Can you work these out from the model? Positions are in its coordinate system, mm. Face numbers are marked on the shaded views. A direction names the side the tool comes from. Give positions to 0.01 mm unless a question says otherwise; leave off trailing zeros. Loops run counter-clockwise (first coordinate to the right, second up) from the corner with the lowest first, then second, coordinate; pieces in that order, holes last. Notation, with made-up numbers: M -26,12.5 L -12,12.5 A26 cw -12,33.5 Z; hole C 22.25,2 d9. An arc over 180 degrees is marked long. Use CSV: the item, a comma, the result in double quotes.
from build123d import *

# Parameters (mm, degrees)
F0_W     = 50
F0_H     = 50
F1_DEPTH = 25
F2_R     = 12.5
F3_DEPTH = 50
F4_R     = 20
F5_DEPTH = 50


with BuildPart() as f1:
    # F0 (on Front) → F1 (new body, symmetric)
    with BuildSketch(Plane.XZ):
        Rectangle(F0_W, F0_H)
    extrude(amount=F1_DEPTH, both=True)

    # F2 (on face) → F3 (cut)
    with BuildSketch(Plane.XZ.offset(25)):
        Circle(F2_R)
    extrude(amount=-F3_DEPTH, mode=Mode.SUBTRACT)

    # F4 (on face) → F5 (join)
    with BuildSketch(Plane.XY.offset(25)):
        Circle(F4_R)
    extrude(amount=F5_DEPTH)

    # F6 (on Front) → F7 (revolve)
    with BuildSketch(Plane.XZ):
        Polygon((0, 103), (0, 75), (10, 75), align=None)
    revolve(axis=Axis((0, 0, 89), (0, 0, 1)))


solid = f1.part
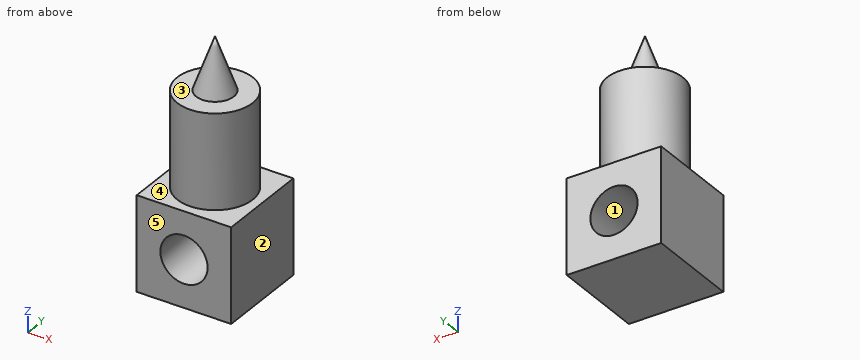
Q1. I want a section at C-C, the plane x = 15. Please give me the cut outline in (y, z).
Model answer:
outline,"M -25,-25 L 25,-25 L 25,25 L 13.23,25 L 13.23,75 L -13.23,75 L -13.23,25 L -25,25 Z"
Q2. If we mould it in two halves opening along Z, with no side actions, what happens to the marked faces 1, 2 and 3? For each: released by +Z, released by -Z, zero draft, split by the parting line, or undercut.
Model answer:
face 1,"undercut"
face 2,"zero draft"
face 3,"released by +Z"
Q3. I'm going to push flat-ended pins straight in: P1, Ø20, axis at x = 7.5, y = 4, coming from the +Z side; P2, Ø4, axis at x = 16, y = -0.5, coming from the +Z side. Where does each tip first touch, or does it pass through?
Model answer:
P1,"z = 103"
P2,"z = 75"
Q4. For the marked faces 4 and 5, which set-ups out of +Z, -Z, +X, -X, +Y, -Y let a thin tool reach every point of the face, with its end or its side?
Model answer:
face 4,"+Z"
face 5,"+Z, -Z, +X, -X, -Y"
Q5. Please list where these lines run through material, in increasing order: L1, parallel to Z at x = -7.5, y = -7; L2, parallel to Z at x = -22, y = -6.5; L3, parallel to Y at x = 0, z = 69.5. Write a range as from..to.
Model answer:
L1,"-25..-10, 10..75"
L2,"-25..25"
L3,"-20..20"
Q6. I want a section at D-D, the plane z = 61. Please give me the cut outline in (x, y), then the cut area to 3 significant figures.
Model answer:
outline,"C 0,0 d40"
area,"1,260 mm2"
Q7. I want a section at B-B, the plane y = 16. Please give me the cut outline in (x, z), then the cut area to 3 significant figures.
Model answer:
outline,"M -25,-25 L 25,-25 L 25,25 L 12,25 L 12,75 L -12,75 L -12,25 L -25,25 Z; hole C 0,0 d25"
area,"3,210 mm2"
Q8. I want a section at A-A, the plane z = 0. Please give me the cut outline in (x, y).
Model answer:
outline,"M -25,-25 L -12.5,-25 L -12.5,25 L -25,25 Z; M 12.5,-25 L 25,-25 L 25,25 L 12.5,25 Z"
